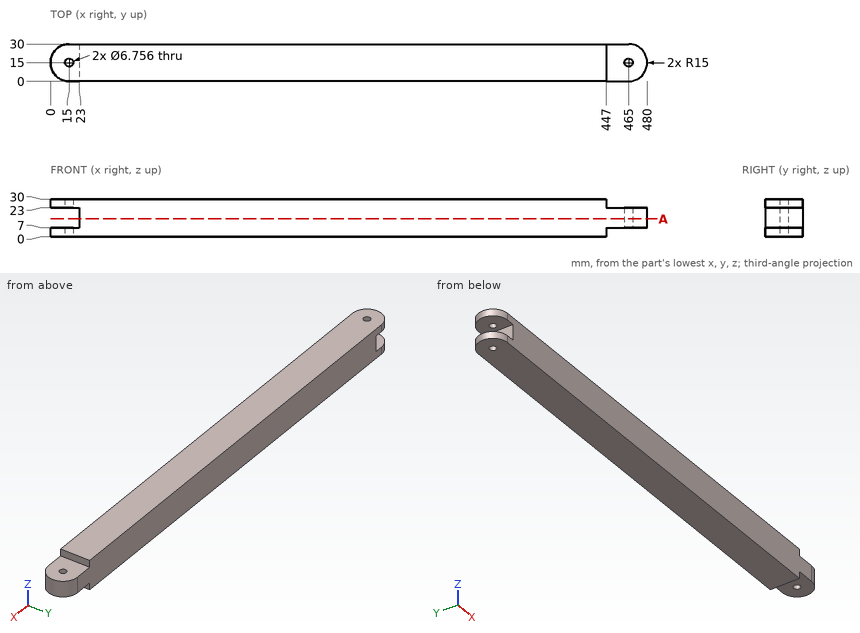
Study the drawing (mm; zero at the part's minimum x, y, z) and answer. Coordinates: 2 decimals unless noted, no trailing zeros. Write each loop counter-clockwise with the first axis right and the second up, starting at its lowest first coordinate (ties: lowest second). Pieces come first, ordered by that corner, then holes.
Q1. Given P1, Ø9, axis at x = 465, y = 15, coming from the -Z side; P2, Ø8, axis at y = 18.5, z = 16.5, coming from the -X side; P3, Ø7.5, axis at y = 20, z = 26.5, coming from the +X side, each flat-ended and moving along its own axis, determine where each tip first touches the part or whether it passes through.
Returned:
P1: stops at z = 7
P2: stops at x = 23
P3: stops at x = 479.55
Q2. Find the intervals of material crossed by line 1 along Y through (x, z) = (15, 25.5); line 2 along Z through (x, y) = (21, 18.5); line 3 along Z through (x, y) = (448.5, 2), in increasing order.
Returned:
line 1: y = 0 to 11.62, 18.38 to 30
line 2: z = 0 to 7, 23 to 30
line 3: z = 7 to 23
Q3. Section A-A, the plane z = 14.25 is taken. Write down the section's boundary in (x, y).
Returned:
outline: (23, 0) - (465, 0) arc R15 ccw to (465, 30) - (23, 30) - close; hole circle Ø6.76 at (465, 15)
